from build123d import *

# Parameters (mm, degrees)
SKETCH1_R           = 3.175
BOSS_EXTRUDE1_DEPTH = 6.35


with BuildPart() as part:
    # Sketch1 → Boss-Extrude1 (new body)
    with BuildSketch(Plane.XY):
        with BuildLine():
            Line((-6.35, 110.49), (-6.35, 0))
            ThreePointArc((-6.35, 0), (0, -6.35), (6.35, 0))
            Line((6.35, 0), (6.35, 110.49))
            Line((6.35, 110.49), (6.35, 180.34))
            Line((6.35, 180.34), (-6.35, 180.34))
            Line((-6.35, 180.34), (-6.35, 110.49))
        make_face()
        with Locations((0, 110.49)):
            Circle(SKETCH1_R, mode=Mode.SUBTRACT)
        Circle(SKETCH1_R, mode=Mode.SUBTRACT)
    extrude(amount=BOSS_EXTRUDE1_DEPTH)


solid = part.part
Geometry: final body of the model. Coordinates: model frame, mm. Give positions to 0.01 mm unless a question says otherwise; leave off trailing zeros. Write each loop counter-clockwise with the first axis right and the second up, starting at its lowest first coordinate (ties: lowest second). Pieces come first, ordered by that corner, then holes. Notation, with made-up numbers: M -10,11.5 L 44,11.5 A28 cw 44,47.5 Z; hole C -16.5,-34 d4. An arc over 180 degrees is marked long. Answer in a Markdown table with one row per item. Add a question column.
(1) Section C-C on z = 4.25. Return loops of the section in (x, y) (3 decimals).
(2) Ray query, line 1 (Y direction, x = 0, z = 3.5) (3 decimals); line 2 (Y direction, x = 2, z = 3.5); line 3 (Y direction, x = 5.5, z = 4.5). Return the intervals inside material, ascending.
(3) First-contact query: pin 1 (3 mm diameter, centred on x = -4, y = 92, fed in from -Z). Flat tip, straight axial feed; report the tip coordinate or a pass-through.
(4) Section A-A on y = 110.49. Return loops of the section in (x, z) (3 decimals).
(5) Mould query, pull axis X, two halves, no side actions, for faces 1 (the cylindrical face through (1.707, 113.167, 3.131)), 2 (the cylindrical face through (-0.69, -3.1, 3.13)), 3 (the flat face through (6.35, 89, 3)), 4 (the flat face through (0, 180.34, 3)). Classes: +X half, -X half, draft (parallel to the pull), parting line (faces both ways), or undercut.
(6) Section B-B on x = 0. Return loops of the section in (y, z) (3 decimals), and give its area (3 significant figures).
Result set:
| question | item | result |
|---|---|---|
| 1 | outline | M -6.35,0 A6.35 ccw 6.35,0 L 6.35,180.34 L -6.35,180.34 Z; hole C 0,0 d6.35; hole C 0,110.49 d6.35 |
| 2 | line 1 | y = -6.35 to -3.175, 3.175 to 107.315, 113.665 to 180.34 |
| 2 | line 2 | y = -6.03 to -2.47, 2.47 to 108.02, 112.96 to 180.34 |
| 2 | line 3 | y = -3.17 to 180.34 |
| 3 | pin 1 | stops at z = 0 |
| 4 | outline | M -6.35,0 L -3.175,0 L -3.175,6.35 L -6.35,6.35 Z; M 3.175,0 L 6.35,0 L 6.35,6.35 L 3.175,6.35 Z |
| 5 | face 1 | undercut |
| 5 | face 2 | undercut |
| 5 | face 3 | +X half |
| 5 | face 4 | draft |
| 6 | outline | M -6.35,0 L -3.175,0 L -3.175,6.35 L -6.35,6.35 Z; M 3.175,0 L 107.315,0 L 107.315,6.35 L 3.175,6.35 Z; M 113.665,0 L 180.34,0 L 180.34,6.35 L 113.665,6.35 Z |
| 6 | area | 1,100 mm^2 |
